Can you work these out from the model? Positions are in its coordinate system, mm. A direction names the side the tool comes from. Give positions to 0.01 mm unless a question says otherwise; leave off trailing zeros. Loops run counter-clockwise (first coordinate to the right, second up) from the corner with the lowest first, then second, coordinate; pieces in that order, holes last. Notation, with made-up numbers: (-21, -8.5) - (28, -8.5) arc R12 ccw to (28, 8.5) - close; hole circle Ø6 at (-6, 67.5). An arc over 180 degrees is marked (long way). Answer in a Markdown table with one row per item.
from build123d import *

# Parameters (mm, degrees)
EXTRUDE_1_DEPTH        = 40
CUT_EXTRUDE_1_REACH    = 122
SKETCH_5_R             = 13
HOLE_WIZARD_M6_1_D     = 5
HOLE_WIZARD_M6_1_DEPTH = 10


with BuildPart() as part:
    # 草图1 → 凸台-拉伸1 (new body)
    with BuildSketch(Plane(origin=(0, 0, 0), x_dir=(0, 0, -1), z_dir=(1, 0, 0))):
        with BuildLine():
            Line((0, 0), (77, 0))
            ThreePointArc((77, 0), (82.656854249, 2.343145751), (85, 8))
            Line((85, 8), (85, 112))
            ThreePointArc((85, 112), (82.656854249, 117.656854249), (77, 120))
            Line((77, 120), (0, 120))
            Line((0, 120), (0, 110))
            Line((0, 110), (67, 110))
            ThreePointArc((67, 110), (72.656854249, 107.656854249), (75, 102))
            Line((75, 102), (75, 18))
            ThreePointArc((75, 18), (72.656854249, 12.343145751), (67, 10))
            Line((67, 10), (0, 10))
            Line((0, 10), (0, 0))
        make_face()
    extrude(amount=EXTRUDE_1_DEPTH)

    # 草图5 → 切除-拉伸1 (cut, up to next)
    with BuildSketch(Plane.XZ, mode=Mode.PRIVATE) as cut_extrude_1_sk1:
        with Locations((20, -35)):
            Circle(SKETCH_5_R)
    cut_extrude_1_tool1 = extrude(cut_extrude_1_sk1.sketch, amount=-CUT_EXTRUDE_1_REACH, mode=Mode.PRIVATE) & part.part
    add(cut_extrude_1_tool1.solids().sort_by_distance((20, 0, -35))[0], mode=Mode.SUBTRACT)

    # M6 螺纹孔1
    with Locations(Plane(origin=(20, 0, -7), x_dir=(0, 0, -1), z_dir=(0, -1, 0))):
        with Locations((0, 0), (56, 0)):
            Hole(HOLE_WIZARD_M6_1_D / 2, depth=HOLE_WIZARD_M6_1_DEPTH)


solid = part.part
Q1. Imagine slicing it at C-C, the plane z = -63. Write out the boundary of the cut face in (x, y).
Checked values:
| item | result |
|---|---|
| outline | (0, 0) - (17.5, 0) - (17.5, 10) - (0, 10) - close; (0, 110) - (40, 110) - (40, 120) - (0, 120) - close; (22.5, 0) - (40, 0) - (40, 10) - (22.5, 10) - close |
Q2. If we mould it in two halves opening along Z, with no side actions, what happens to faces 1 (the face through (19.72, 2.281, -82.594)), 2 (the face through (32.4, 4.9, -31.1)), 3 (the face through (20, 115, 0)), 4 (the face through (22.11, 5.07, -61.66))? For each: released by +Z, released by -Z, zero draft, split by the parting line, or undercut.
Checked values:
| item | result |
|---|---|
| face 1 | released by -Z |
| face 2 | undercut |
| face 3 | released by +Z |
| face 4 | undercut |
Q3. On a 3-axis mill with a long thin cutter (end or side, diameter ignored), from which of +Z, -Z, +X, -X, +Y, -Y can I reach the whole of each face in a straight line? I mean faces 5 (the face through (22.11, 5.07, -5.66)), 6 (the face through (20, 5, 0)), 7 (the face through (19.72, 12.406, -72.719)). Say none if no direction works.
Checked values:
| item | result |
|---|---|
| face 5 | -Y |
| face 6 | +Z, +X, -X, +Y, -Y |
| face 7 | +Z, +X, -X |
Q4. Imagine slicing it at D-D, the plane x = 36. Write out the boundary of the cut face in (y, z), and give its area (3 significant figures).
Checked values:
| item | result |
|---|---|
| outline | (0, -77) arc R8 ccw to (8, -85) - (112, -85) arc R8 ccw to (120, -77) - (120, 0) - (110, 0) - (110, -67) arc R8 cw to (102, -75) - (18, -75) arc R8 cw to (10, -67) - (10, 0) - (0, 0) - close |
| area | 2,700 mm² |
Q5. Imagine slicing it at B-B, the plane z = -14.5. Write out the boundary of the cut face in (x, y).
Checked values:
| item | result |
|---|---|
| outline | (0, 0) - (40, 0) - (40, 10) - (0, 10) - close; (0, 110) - (40, 110) - (40, 120) - (0, 120) - close |
Q6. If I drill on line 1 (X direction, y = 3, z = -63); line 2 (Y direction, x = 5, z = -23); line 3 (Z direction, x = 21, y = 80), over which ranges is the centre line in solid material (lowest first)? Write a range as [from, to].
Checked values:
| item | result |
|---|---|
| line 1 | x = [0, 17.5], [22.5, 40] |
| line 2 | y = [0, 10], [110, 120] |
| line 3 | z = [-85, -75] |
Q7. Imagine slicing it at A-A, the plane x = 25. Write out the boundary of the cut face in (y, z).
Checked values:
| item | result |
|---|---|
| outline | (0, -77) arc R8 ccw to (8, -85) - (112, -85) arc R8 ccw to (120, -77) - (120, 0) - (110, 0) - (110, -67) arc R8 cw to (102, -75) - (18, -75) arc R8 cw to (10, -67) - (10, -47) - (0, -47) - close; (0, -23) - (10, -23) - (10, 0) - (0, 0) - close |
Q8. For pin 1 (20 mm diameter, centred on x = 11, y = 50, fed in from +Z); pin 2 (3 mm diameter, centred on x = 20, z = -63, fed in from -Y), each with a flat end and sliding along its axis, tell me the tip position at first contact or that it passes through.
Checked values:
| item | result |
|---|---|
| pin 1 | stops at z = -75 |
| pin 2 | stops at y = 110 |
